```python
from build123d import *

# Parameters (mm, degrees)
SKETCH017_R  = 6.9
PAD007_DEPTH = 20


with BuildPart() as part:
    # Sketch017 → Pad007 (new body, symmetric)
    with BuildSketch(Plane.XZ.offset(-200)):
        with BuildLine():
            ThreePointArc((21, 40.7), (11, 30.7), (21, 20.7))
            ThreePointArc((31, 10.7), (28.071068, 17.771068), (21, 20.7))
            Line((37.9, 10.7), (31, 10.7))
            Line((37.9, 50.7), (37.9, 10.7))
            Line((31, 50.7), (37.9, 50.7))
            ThreePointArc((21, 40.7), (28.071068, 43.628932), (31, 50.7))
        make_face()
        with Locations((21, 30.7)):
            Circle(SKETCH017_R, mode=Mode.SUBTRACT)
    extrude(amount=PAD007_DEPTH, both=True)


solid = part.part
```
Input: part model. Units: mm. Frame: model coordinates. Coordinates: 2 decimals unless noted, no trailing zeros. Order: outer loops, then holes, each group sorted by start corner. A loop starts at its lowest first (then second) coordinate and runs counter-clockwise, first axis right, second up. Notation, with made-up numbers: (38, -26.5) - (91, -26.5) arc R17 cw to (91, -16.5) - close; hole circle Ø3 at (64.25, 8.5). An arc over 180 degrees is marked (long way). Return JSON: item names as keys, results as strings.
Q1. Cut plane B-B (x = 17.5). Return loops of the section in (y, z), then the cut area to 3 significant figures.
The answers:
{"outline": "(180, 21.33) - (220, 21.33) - (220, 24.75) - (180, 24.75) - close; (180, 36.65) - (220, 36.65) - (220, 40.07) - (180, 40.07) - close", "area": "274 mm2"}
Q2. First-contact query: pin 1 (6 mm diameter, centred on x = 22, y = 214, fed in from +Z); pin 2 (2 mm diameter, centred on x = 14, y = 213, fed in from -Z); pin 3 (8 mm diameter, centred on y = 201, z = 17.5, fed in from -X). Flat tips, straight axial feed; report the tip coordinate or a pass-through.
The answers:
{"pin 1": "stops at z = 41.53", "pin 2": "stops at z = 22.7", "pin 3": "stops at x = 17.08"}
Q3. Cut plane C-C (z = 30.7). Return loops of the section in (x, y), then the cut area to 3 significant figures.
The answers:
{"outline": "(11, 180) - (14.1, 180) - (14.1, 220) - (11, 220) - close; (27.9, 180) - (37.9, 180) - (37.9, 220) - (27.9, 220) - close", "area": "524 mm2"}
Q4. Cut plane D-D (z = 40). Return loops of the section in (x, y), then the cut area to 3 significant figures.
The answers:
{"outline": "(17.32, 180) - (37.9, 180) - (37.9, 220) - (17.32, 220) - close", "area": "823 mm2"}
Q5. Cut plane A-A (y = 192.5). Return loops of the section in (x, z).
The answers:
{"outline": "(21, 20.7) arc R10 cw to (31, 10.7) - (37.9, 10.7) - (37.9, 50.7) - (31, 50.7) arc R10 cw to (21, 40.7) arc R10 ccw to start; hole circle Ø13.8 at (21, 30.7)"}
Q6. Ray query, probe 1 along X at (y, z) = (186.5, 31); probe 2 along Z at (x, y) = (21, 200); probe 3 along X at (y, z) = (202, 34.5). Return the intervals inside material, ascending.
The answers:
{"probe 1": "x = 11 to 14.11, 27.89 to 37.9", "probe 2": "z = 20.7 to 23.8, 37.6 to 40.7", "probe 3": "x = 11.75 to 15.24, 26.76 to 37.9"}
